from build123d import *

# Parameters (mm, degrees)
ESQUISSE2_W        = 46.2
ESQUISSE2_H        = 5
ESQUISSE2_H_2      = 8
ESQUISSE2_H_3      = 8.88649877
ESQUISSE2_H_4      = 2
ESQUISSE2_H_5      = 4.567327767
BOSS_EXTRU_1_DEPTH = 5
ESQUISSE3_W        = 46.2
ESQUISSE3_H        = 25.11350123
ESQUISSE3_H_2      = 26
BOSS_EXTRU_2_DEPTH = 3


with BuildPart() as part:
    # Esquisse2 → Boss.-Extru.1 (new body)
    with BuildSketch(Plane(origin=(0, 0, 0), x_dir=(1, 0, 0), z_dir=(0, 1, 0))):
        with BuildLine():
            Line((-75.44494324, 137.861939651), (-85.44494324, 137.861939651))
            Line((-85.44494324, 137.861939651), (-85.44494324, 127.861939651))
            Line((-85.44494324, 127.861939651), (-77.44494324, 127.861939651))
            ThreePointArc((-77.44494324, 127.861939651), (-76.859156802, 129.276153213), (-75.44494324, 129.861939651))
            Line((-75.44494324, 129.861939651), (-75.44494324, 137.861939651))
        make_face()
        with BuildLine():
            Line((-77.44494324, 127.861939651), (-85.44494324, 127.861939651))
            Line((-85.44494324, 127.861939651), (-85.44494324, -39.841561579))
            Line((-85.44494324, -39.841561579), (-77.44494324, -39.841561579))
            ThreePointArc((-77.44494324, -39.841561579), (-76.859156802, -38.427348016), (-75.44494324, -37.841561579))
            Line((-75.44494324, -37.841561579), (-75.44494324, 125.861939651))
            ThreePointArc((-75.44494324, 125.861939651), (-76.859156802, 126.447726088), (-77.44494324, 127.861939651))
        make_face()
        with BuildLine():
            Line((-70.44494324, 127.861939651), (-73.44494324, 127.861939651))
            ThreePointArc((-73.44494324, 127.861939651), (-74.030729678, 126.447726088), (-75.44494324, 125.861939651))
            Line((-75.44494324, 125.861939651), (-75.44494324, -37.841561579))
            ThreePointArc((-75.44494324, -37.841561579), (-74.030729678, -38.427348016), (-73.44494324, -39.841561579))
            Line((-73.44494324, -39.841561579), (-70.44494324, -39.841561579))
            Line((-70.44494324, -39.841561579), (-70.44494324, 127.861939651))
        make_face()
        with BuildLine():
            Line((118.43505676, 101.861939651), (118.43505676, 127.861939651))
            Line((118.43505676, 127.861939651), (-43.44494324, 127.861939651))
            ThreePointArc((-43.44494324, 127.861939651), (-45.44494324, 125.861939651), (-47.44494324, 127.861939651))
            Line((-47.44494324, 127.861939651), (-70.44494324, 127.861939651))
            Line((-70.44494324, 127.861939651), (-70.44494324, -39.841561579))
            Line((-70.44494324, -39.841561579), (-47.44494324, -39.841561579))
            ThreePointArc((-47.44494324, -39.841561579), (-45.44494324, -37.841561579), (-43.44494324, -39.841561579))
            Line((-43.44494324, -39.841561579), (118.43505676, -39.841561579))
            Line((118.43505676, -39.841561579), (118.43505676, -35.312608687))
            Line((118.43505676, -35.312608687), (118.43505676, -14.728060349))
            Line((118.43505676, -14.728060349), (118.43505676, -10.160732582))
            Line((118.43505676, -10.160732582), (118.43505676, 33.566939651))
            Line((118.43505676, 33.566939651), (118.43505676, 37.839267418))
            Line((118.43505676, 37.839267418), (118.43505676, 48.861939651))
            Line((118.43505676, 48.861939651), (118.43505676, 53.566939651))
            Line((118.43505676, 53.566939651), (118.43505676, 96.861939651))
            Line((118.43505676, 96.861939651), (118.43505676, 101.861939651))
        make_face()
        with BuildLine():
            Line((-77.44494324, -39.841561579), (-85.44494324, -39.841561579))
            Line((-85.44494324, -39.841561579), (-85.44494324, -50.728060349))
            Line((-85.44494324, -50.728060349), (-75.44494324, -50.728060349))
            Line((-75.44494324, -50.728060349), (-75.44494324, -41.841561579))
            ThreePointArc((-75.44494324, -41.841561579), (-76.859156802, -41.255775141), (-77.44494324, -39.841561579))
        make_face()
        with BuildLine():
            Line((-75.44494324, -41.841561579), (-75.44494324, -50.728060349))
            Line((-75.44494324, -50.728060349), (118.43505676, -50.728060349))
            Line((118.43505676, -50.728060349), (118.43505676, -48.728060349))
            Line((118.43505676, -48.728060349), (118.43505676, -39.841561579))
            Line((118.43505676, -39.841561579), (-43.44494324, -39.841561579))
            ThreePointArc((-43.44494324, -39.841561579), (-45.44494324, -41.841561579), (-47.44494324, -39.841561579))
            Line((-47.44494324, -39.841561579), (-70.44494324, -39.841561579))
            Line((-70.44494324, -39.841561579), (-73.44494324, -39.841561579))
            ThreePointArc((-73.44494324, -39.841561579), (-74.030729678, -41.255775141), (-75.44494324, -41.841561579))
        make_face()
        with BuildLine():
            Line((349.300456076, 127.861939651), (164.63505676, 127.861939651))
            Line((164.63505676, 127.861939651), (164.63505676, 101.861939651))
            Line((164.63505676, 101.861939651), (164.63505676, 96.861939651))
            Line((164.63505676, 96.861939651), (189.43505676, 96.861939651))
            Line((189.43505676, 96.861939651), (189.43505676, 48.861939651))
            Line((189.43505676, 48.861939651), (164.63505676, 48.861939651))
            Line((164.63505676, 48.861939651), (164.63505676, 43.566939651))
            Line((164.63505676, 43.566939651), (164.63505676, 37.839267418))
            Line((164.63505676, 37.839267418), (189.43505676, 37.839267418))
            Line((189.43505676, 37.839267418), (189.43505676, -10.160732582))
            Line((189.43505676, -10.160732582), (164.63505676, -10.160732582))
            Line((164.63505676, -10.160732582), (164.63505676, -14.728060349))
            Line((164.63505676, -14.728060349), (164.63505676, -39.841561579))
            Line((164.63505676, -39.841561579), (349.300456076, -39.841561579))
            ThreePointArc((349.300456076, -39.841561579), (351.300456076, -37.841561579), (353.300456076, -39.841561579))
            Line((353.300456076, -39.841561579), (377.70505676, -39.841561579))
            Line((377.70505676, -39.841561579), (377.70505676, 127.861939651))
            Line((377.70505676, 127.861939651), (353.300456076, 127.861939651))
            ThreePointArc((353.300456076, 127.861939651), (351.300456076, 125.861939651), (349.300456076, 127.861939651))
        make_face()
        with BuildLine():
            Line((381.300456076, 137.861939651), (118.43505676, 137.861939651))
            Line((118.43505676, 137.861939651), (118.43505676, 135.861939651))
            Line((118.43505676, 135.861939651), (164.63505676, 135.861939651))
            Line((164.63505676, 135.861939651), (164.63505676, 127.861939651))
            Line((164.63505676, 127.861939651), (349.300456076, 127.861939651))
            ThreePointArc((349.300456076, 127.861939651), (351.300456076, 129.861939651), (353.300456076, 127.861939651))
            Line((353.300456076, 127.861939651), (377.70505676, 127.861939651))
            Line((377.70505676, 127.861939651), (379.300456076, 127.861939651))
            ThreePointArc((379.300456076, 127.861939651), (379.886242514, 129.276153213), (381.300456076, 129.861939651))
            Line((381.300456076, 129.861939651), (381.300456076, 137.861939651))
        make_face()
        with BuildLine():
            Line((392.70505676, -39.841561579), (392.70505676, 127.861939651))
            Line((392.70505676, 127.861939651), (383.300456076, 127.861939651))
            ThreePointArc((383.300456076, 127.861939651), (382.714669639, 126.447726088), (381.300456076, 125.861939651))
            Line((381.300456076, 125.861939651), (381.300456076, -37.841561579))
            ThreePointArc((381.300456076, -37.841561579), (382.714669639, -38.427348016), (383.300456076, -39.841561579))
            Line((383.300456076, -39.841561579), (392.70505676, -39.841561579))
        make_face()
        with BuildLine():
            Line((392.70505676, 137.861939651), (381.300456076, 137.861939651))
            Line((381.300456076, 137.861939651), (381.300456076, 129.861939651))
            ThreePointArc((381.300456076, 129.861939651), (382.714669639, 129.276153213), (383.300456076, 127.861939651))
            Line((383.300456076, 127.861939651), (392.70505676, 127.861939651))
            Line((392.70505676, 127.861939651), (392.70505676, 137.861939651))
        make_face()
        Polygon((164.63505676, 48.861939651), (118.43505676, 48.861939651), (118.43505676, 37.839267418), (164.63505676, 37.839267418), (164.63505676, 43.566939651), align=None)
        with Locations((141.53505676, 99.361939651)):
            Rectangle(ESQUISSE2_W, ESQUISSE2_H)
        with Locations((141.53505676, 131.861939651)):
            Rectangle(ESQUISSE2_W, ESQUISSE2_H_2)
        with BuildLine():
            Line((118.43505676, 137.861939651), (-75.44494324, 137.861939651))
            Line((-75.44494324, 137.861939651), (-75.44494324, 129.861939651))
            ThreePointArc((-75.44494324, 129.861939651), (-74.030729678, 129.276153213), (-73.44494324, 127.861939651))
            Line((-73.44494324, 127.861939651), (-70.44494324, 127.861939651))
            Line((-70.44494324, 127.861939651), (-47.44494324, 127.861939651))
            ThreePointArc((-47.44494324, 127.861939651), (-45.44494324, 129.861939651), (-43.44494324, 127.861939651))
            Line((-43.44494324, 127.861939651), (118.43505676, 127.861939651))
            Line((118.43505676, 127.861939651), (118.43505676, 135.861939651))
            Line((118.43505676, 135.861939651), (118.43505676, 137.861939651))
        make_face()
        with Locations((141.53505676, -44.284810964)):
            Rectangle(ESQUISSE2_W, ESQUISSE2_H_3)
        with Locations((141.53505676, -49.728060349)):
            Rectangle(ESQUISSE2_W, ESQUISSE2_H_4)
        with BuildLine():
            Line((164.63505676, -48.728060349), (164.63505676, -50.728060349))
            Line((164.63505676, -50.728060349), (377.70505676, -50.728060349))
            Line((377.70505676, -50.728060349), (377.70505676, -39.841561579))
            Line((377.70505676, -39.841561579), (353.300456076, -39.841561579))
            ThreePointArc((353.300456076, -39.841561579), (351.300456076, -41.841561579), (349.300456076, -39.841561579))
            Line((349.300456076, -39.841561579), (164.63505676, -39.841561579))
            Line((164.63505676, -39.841561579), (164.63505676, -48.728060349))
        make_face()
        with Locations((141.53505676, -12.444396466)):
            Rectangle(ESQUISSE2_W, ESQUISSE2_H_5)
        with BuildLine():
            Line((379.300456076, -39.841561579), (377.70505676, -39.841561579))
            Line((377.70505676, -39.841561579), (377.70505676, -50.728060349))
            Line((377.70505676, -50.728060349), (381.300456076, -50.728060349))
            Line((381.300456076, -50.728060349), (381.300456076, -41.841561579))
            ThreePointArc((381.300456076, -41.841561579), (379.886242514, -41.255775141), (379.300456076, -39.841561579))
        make_face()
        with BuildLine():
            Line((392.70505676, -50.728060349), (392.70505676, -39.841561579))
            Line((392.70505676, -39.841561579), (383.300456076, -39.841561579))
            ThreePointArc((383.300456076, -39.841561579), (382.714669639, -41.255775141), (381.300456076, -41.841561579))
            Line((381.300456076, -41.841561579), (381.300456076, -50.728060349))
            Line((381.300456076, -50.728060349), (392.70505676, -50.728060349))
        make_face()
        with BuildLine():
            ThreePointArc((381.300456076, 125.861939651), (379.886242514, 126.447726088), (379.300456076, 127.861939651))
            Line((379.300456076, 127.861939651), (377.70505676, 127.861939651))
            Line((377.70505676, 127.861939651), (377.70505676, -39.841561579))
            Line((377.70505676, -39.841561579), (379.300456076, -39.841561579))
            ThreePointArc((379.300456076, -39.841561579), (379.886242514, -38.427348016), (381.300456076, -37.841561579))
            Line((381.300456076, -37.841561579), (381.300456076, 125.861939651))
        make_face()
    extrude(amount=BOSS_EXTRU_1_DEPTH)

    # Esquisse3 → Boss.-Extru.2 (add)
    with BuildSketch(Plane.XZ):
        with Locations((141.53505676, 27.284810964)):
            Rectangle(ESQUISSE3_W, ESQUISSE3_H)
        with Locations((141.53505676, -114.861939651)):
            Rectangle(ESQUISSE3_W, ESQUISSE3_H_2)
    extrude(amount=-BOSS_EXTRU_2_DEPTH)


solid = part.part
Design review of the part built by this model. Coordinates are the model's own, in mm. Give positions to 0.01 mm unless a question says otherwise; leave off trailing zeros. Order: outer loops, then holes, each group sorted by start corner. A loop starts at its lowest first (then second) coordinate and runs counter-clockwise, first axis right, second up. Notation, with made-up numbers: (56.5, 9.25) - (74.5, 9.25) arc R20 cw to (74.5, 28.25) - close; hole circle Ø11 at (72, -28). An arc over 180 degrees is marked (long way). Use CSV: the item, a comma, the result in double quotes. Start each with the question number.
Q1. Draft analysis for pull direction Z (two halves, no side actions). For faces 1 (the face through (141, 3, -115)), 2 (the face through (141, 3, 27)), 3 (the face through (150, 5, -45)), state which applies: pulls with the +Z half, pulls with the -Z half, needs draft (parallel to the pull), parting line crosses it, or undercut.
Q2. For line 1 (Z direction, x = 123.5, y = 2.65); line 2 (X direction, y = 3.4, z = 39.5); line 3 (X direction, y = 3.1, z = -76.5), list the stretches that pass through material, from the lowest coordinate up.
Q3. For P1, Ø13, axis at x = 133.5, z = -120.5, coming from the +Y side, flat-tipped, find the tip position at first contact; note if it passes through.
Q4. Take a section at A-A (z = -8). State the section outline as (x, y) points.
Q5. Take a section at B-B (y = 1.45). Count the separate pieces of the cut face and the enclosed holes in it, and give its area (3 significant figures).
Q6. Take a section at C-C (z = 31.5). State the section outline as (x, y) points.
Calculated:
1,face 1,"undercut"
1,face 2,"undercut"
1,face 3,"needs draft"
2,line 1,"z = -137.86 to -96.86, -48.86 to -37.84, 10.16 to 50.73"
2,line 2,"x = -85.44 to -77.42, -73.47 to -47.42, -43.47 to 118.44, 164.64 to 349.33, 353.27 to 379.33, 383.27 to 392.71"
2,line 3,"x = -85.44 to 118.44, 189.44 to 392.71"
3,P1,"stops at y = 3"
4,outline,"(-85.44, 0) - (118.44, 0) - (118.44, 5) - (-85.44, 5) - close; (189.44, 0) - (392.71, 0) - (392.71, 5) - (189.44, 5) - close"
5,separate pieces,"1"
5,enclosed holes,"10"
5,area,"83,300 mm²"
6,outline,"(-85.44, 0) - (392.71, 0) - (392.71, 5) - (164.64, 5) - (164.64, 3) - (118.44, 3) - (118.44, 5) - (-85.44, 5) - close"
